Study the drawing (mm; zero at the part's minimum x, y, z) and answer. A direction names the side the tool comes from. Coordinates: 2 decimals unless noted, no trailing zeros. Order: outer loops, then holes, each group sorted by start corner. A loop starts at its lowest first (then second) coordinate and runs counter-clockwise, first axis right, second up. Notation, with made-up numbers: M 87.5,18.5 L 126.5,18.5 A15 cw 126.5,41.5 Z; hole C 43.25,74.25 d10. An arc over 180 degrees is marked long. One line per item, written item: value. Start each with the question number.
Q1. The part is cut by section C-C on y = 43.5. Give the vertices of the cut face in (x, z), then the cut area to 3 significant figures.
Q2. Each of these flat-tipped pins is pushed along its axis until it touches: pin 1 Ø12 at (y, z) = (42, 29.5) entering from +X; pin 2 Ø2 at (y, z) = (66.5, 33.5) entering from +X; pin 3 Ø5 at (x, y) = (76.5, 57) entering from +Z. Where does it stop, or does it pass through?
Q3. Straight lines are drawn through the part: line 1 along X through (y, z) = (25, 49) (1 decimal); line 2 along X through (y, z) = (14.5, 35.5) (1 decimal); line 3 along Z through (x, y) = (69, 5). For each, find the intervals that lie inside material, in ascending order. Write a range as [from, to].
Q4. Determine the mould class of the marked faces 3, 4 and 5 for opening direction X: pulls with the +X half, pulls with the -X half, needs draft (parallel to the pull), parting line crosses it, or undercut.
Q5. For the marked faces 1 and 2, determine the directions among +Z, -Z, +X, -X, +Y, -Y from which every point of the face is accessible in a straight line to the end or side of a thin tool.
Q6. The part is cut by section D-D on y = 18. Give the vertices of the cut face in (x, z), then the cut area to 3 significant figures.
Q7. The part is cut by section B-B on x = 56. Give the vertices of the cut face in (y, z), then the cut area to 3 significant figures.
Q8. The part is cut by section A-A on z = 36. Give the vertices of the cut face in (x, y), then the cut area to 3 significant figures.
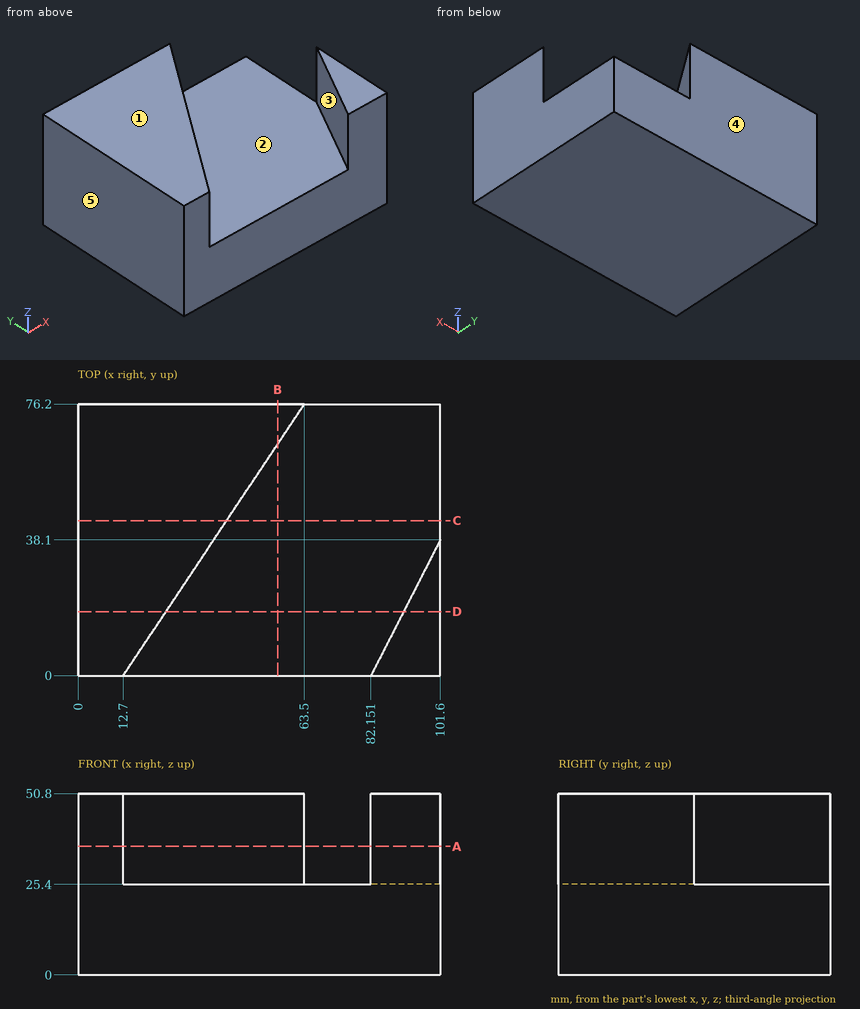
Output:
1. outline: M 0,0 L 101.6,0 L 101.6,25.4 L 41.7,25.4 L 41.7,50.8 L 0,50.8 Z
1. area: 3,640 mm^2
2. pin 1: stops at x = 101.6
2. pin 2: stops at x = 57.7
2. pin 3: stops at z = 25.4
3. line 1: x = [0, 29.4], [94.9, 101.6]
3. line 2: x = [0, 22.4], [89.6, 101.6]
3. line 3: z = [0, 25.4]
4. face 3: undercut
4. face 4: needs draft
4. face 5: pulls with the -X half
5. face 1: +Z, +X, -X, +Y, -Y
5. face 2: +Z
6. outline: M 0,0 L 101.6,0 L 101.6,50.8 L 91.34,50.8 L 91.34,25.4 L 24.7,25.4 L 24.7,50.8 L 0,50.8 Z
6. area: 3,470 mm^2
7. outline: M 0,0 L 76.2,0 L 76.2,50.8 L 64.95,50.8 L 64.95,25.4 L 0,25.4 Z
7. area: 2,220 mm^2
8. outline: M 0,0 L 12.7,0 L 63.5,76.2 L 0,76.2 Z; M 82.15,0 L 101.6,0 L 101.6,38.1 Z
8. area: 3,270 mm^2
